from build123d import *

# Parameters (mm, degrees)
SKETCH1_R           = 2.9337
BOSS_EXTRUDE1_DEPTH = 63.5


with BuildPart() as part:
    # Sketch1 → Boss-Extrude1 (new body)
    with BuildSketch(Plane(origin=(0, 0, 0), x_dir=(-1, 0, 0), z_dir=(0, 0, -1))):
        with BuildLine():
            Line((-7.332348419, 4.44e-07), (-6.293011423, -1.80018429))
            ThreePointArc((-6.293011423, -1.80018429), (-4.12444613, -2.38124975), (-4.70551159, -4.549815043))
            Line((-4.70551159, -4.549815043), (-3.666174594, -6.349999778))
            Line((-3.666174594, -6.349999778), (-1.587500385, -6.349999778))
            ThreePointArc((-1.587500385, -6.349999778), (-3.85e-07, -4.762499778), (1.587499615, -6.349999778))
            Line((1.587499615, -6.349999778), (3.666173825, -6.349999778))
            Line((3.666173825, -6.349999778), (4.705510929, -4.549815106))
            ThreePointArc((4.705510929, -4.549815106), (4.124445601, -2.381249778), (6.293010929, -1.800184449))
            Line((6.293010929, -1.800184449), (7.332348034, 2.22e-07))
            Line((7.332348034, 2.22e-07), (6.293011189, 1.800184821))
            ThreePointArc((6.293011189, 1.800184821), (4.124445913, 2.381250347), (4.705511439, 4.549815623))
            Line((4.705511439, 4.549815623), (3.666174594, 6.350000222))
            Line((3.666174594, 6.350000222), (1.587500385, 6.350000222))
            ThreePointArc((1.587500385, 6.350000222), (3.85e-07, 4.762500222), (-1.587499615, 6.350000222))
            Line((-1.587499615, 6.350000222), (-3.666173825, 6.350000222))
            Line((-3.666173825, 6.350000222), (-4.705511038, 4.549815614))
            ThreePointArc((-4.705511038, 4.549815614), (-4.124445841, 2.38125025), (-6.293011205, 1.800185053))
            Line((-6.293011205, 1.800185053), (-7.332348419, 4.44e-07))
        make_face()
        Circle(SKETCH1_R, mode=Mode.SUBTRACT)
    extrude(amount=-BOSS_EXTRUDE1_DEPTH)


solid = part.part
Verification items for the finished model (mm, model axes). Give positions to 0.01 mm unless a question says otherwise; leave off trailing zeros. Write each loop counter-clockwise with the first axis right and the second up, starting at its lowest first coordinate (ties: lowest second). Pieces come first, ordered by that corner, then holes.
(1) Gauge pin test, flat ends, axial feed: pin 1 (1.5 mm diameter, centred on y = 2, z = 37, fed in from -X); pin 2 (1 mm diameter, centred on y = 2, z = 26, fed in from -X). Record the tip position at first contact, or that the pin passes through.
(2) Cross-section at B-B (x = 0). Enter the section's corners in (y, z).
(3) Material ranges on line 1 (Y direction, x = 0, z = 15); line 2 (X direction, y = -3, z = 7); line 3 (X direction, y = 0.75, z = 4), recorded low to high.
(4) Mould release check, pull along Y, two halves, no side actions. Record for faces 1 (the face through (6.82, -0.89, 31.31)), 2 (the face through (4.11, 2.41, 31.31)), 3 (the face through (4.18, 5.46, 31.31)): +Y half, -Y half, draft (parallel to the pull), parting line (faces both ways), or undercut.
Worked out:
1. pin 1: stops at x = -6.61
1. pin 2: stops at x = -6.47
2. outline: (-4.76, 0) - (-2.93, 0) - (-2.93, 63.5) - (-4.76, 63.5) - close; (2.93, 0) - (4.76, 0) - (4.76, 63.5) - (2.93, 63.5) - close
3. line 1: y = -4.76 to -2.93, 2.93 to 4.76
3. line 2: x = -3.92 to 3.92
3. line 3: x = -6.9 to -2.84, 2.84 to 6.9
4. face 1: -Y half
4. face 2: undercut
4. face 3: +Y half
